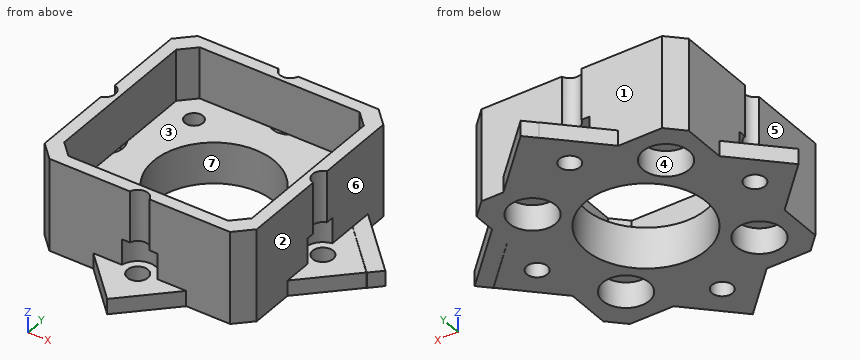
from build123d import *

# Parameters (mm, degrees)
F4_DEPTH  = 18
F2_R      = 1.75
F2_R_2    = 11.75
F5_DEPTH  = 8
F3_R      = 2
F3_R_2    = 1.75
F3_R_3    = 11.75
F6_DEPTH  = 3
F7_DEPTH  = 18
F8_R      = 4.5
F8_R_2    = 1.75
F9_DEPTH  = 5
F10_DEPTH = 5
F11_R     = 3.5
F12_DEPTH = 5
F14_DEPTH = 3
F15_DEPTH = 5
F16_DEPTH = 5
F17_R     = 1.75
F18_DEPTH = 5


with BuildPart() as f4:
    # F1 (on Top) → F4 (new body)
    with BuildSketch(Plane.XY):
        Polygon((-17.5979303911, 20.6482383256), (-20.6482383256, 17.5979303911), (-20.6482383256, -17.5979303911), (-17.5979303911, -20.6482383256), (17.5979303911, -20.6482383256), (20.6482383256, -17.5979303911), (20.6482383256, 17.5979303911), (17.5979303911, 20.6482383256), align=None)
        Polygon((-15.5676494429, -18.266042013), (-18.266042013, -15.5676494429), (-18.266042013, 15.5676494429), (-15.5676494429, 18.266042013), (15.5676494429, 18.266042013), (18.266042013, 15.5676494429), (18.266042013, -15.5676494429), (15.5676494429, -18.266042013), align=None, mode=Mode.SUBTRACT)
    extrude(amount=F4_DEPTH)

    # F2 (on Top) → F5 (join)
    with BuildSketch(Plane.XY):
        Polygon((-15.5676494429, 18.266042013), (-18.266042013, 15.5676494429), (-18.266042013, -15.5676494429), (-15.5676494429, -18.266042013), (15.5676494429, -18.266042013), (18.266042013, -15.5676494429), (18.266042013, 15.5676494429), (15.5676494429, 18.266042013), align=None)
        with Locations((-13, -13)):
            Circle(F2_R, mode=Mode.SUBTRACT)
        with Locations((13, -13)):
            Circle(F2_R, mode=Mode.SUBTRACT)
        with Locations((-13, 13)):
            Circle(F2_R, mode=Mode.SUBTRACT)
        Circle(F2_R_2, mode=Mode.SUBTRACT)
        with Locations((13, 13)):
            Circle(F2_R, mode=Mode.SUBTRACT)
    extrude(amount=F5_DEPTH)

    # F3 (on Top) → F6 (join)
    with BuildSketch(Plane.XY):
        Polygon((-29.6984848098, 0), (0, -29.6984848098), (29.6984848098, 0), (0, 29.6984848098), align=None)
        with Locations((0, -21.2132034356)):
            Circle(F3_R, mode=Mode.SUBTRACT)
        with Locations((-13, -13)):
            Circle(F3_R_2, mode=Mode.SUBTRACT)
        with Locations((13, -13)):
            Circle(F3_R_2, mode=Mode.SUBTRACT)
        with Locations((-21.2132034356, 0)):
            Circle(F3_R, mode=Mode.SUBTRACT)
        Circle(F3_R_3, mode=Mode.SUBTRACT)
        with Locations((-13, 13)):
            Circle(F3_R_2, mode=Mode.SUBTRACT)
        with Locations((0, 21.2132034356)):
            Circle(F3_R, mode=Mode.SUBTRACT)
        with Locations((13, 13)):
            Circle(F3_R_2, mode=Mode.SUBTRACT)
        with Locations((21.2132034356, 0)):
            Circle(F3_R, mode=Mode.SUBTRACT)
    extrude(amount=F6_DEPTH)

    # F3 (on Top) → F7 (cut)
    with BuildSketch(Plane.XY):
        with Locations((21.2132034356, 0)):
            Circle(F3_R)
        with Locations((0, 21.2132034356)):
            Circle(F3_R)
        with Locations((0, -21.2132034356)):
            Circle(F3_R)
        with Locations((-21.2132034356, 0)):
            Circle(F3_R)
    extrude(amount=F7_DEPTH, mode=Mode.SUBTRACT)

    # F8 (on face) + F2 (on Top) → F9 (cut)
    with BuildSketch(Plane(origin=(0, 0, 0), x_dir=(1, 0, 0), z_dir=(0, 0, -1))):
        with Locations((-13, -13)):
            Circle(F8_R)
        with Locations((-13, -13)):
            Circle(F8_R_2, mode=Mode.SUBTRACT)
    with BuildSketch(Plane.XY):
        with Locations((-13, 13)):
            Circle(F2_R)
    extrude(amount=-F9_DEPTH, dir=(0, 0, -1), mode=Mode.SUBTRACT)

    # F8 (on face) + F2 (on Top) → F10 (cut)
    with BuildSketch(Plane(origin=(0, 0, 0), x_dir=(1, 0, 0), z_dir=(0, 0, -1))):
        with Locations((13, 13)):
            Circle(F8_R)
        with Locations((13, 13)):
            Circle(F8_R_2, mode=Mode.SUBTRACT)
    with BuildSketch(Plane.XY):
        with Locations((13, -13)):
            Circle(F2_R)
    extrude(amount=-F10_DEPTH, dir=(0, 0, -1), mode=Mode.SUBTRACT)

    # F11 (on face) → F12 (cut)
    with BuildSketch(Plane.XY.offset(3)):
        with Locations((0, 21.2132034356)):
            Circle(F11_R)
        with Locations((0, -21.2132034356)):
            Circle(F11_R)
        with Locations((21.2132034356, 0)):
            Circle(F11_R)
        with Locations((-21.2132034356, 0)):
            Circle(F11_R)
    extrude(amount=F12_DEPTH, mode=Mode.SUBTRACT)

    # F13 (on face) → F14 (join)
    with BuildSketch(Plane.XY):
        Polygon((13.4627325878, 20.5004686409), (2.1524152157, 31.7889230696), (0.030988478, 29.6674963319), (9.1980161689, 20.5004686409), align=None)
        Polygon((31.875104401, 2.1236881052), (20.4795914376, 13.4971734413), (20.4795914376, 9.2360144303), (29.7514162958, 0), align=None)
    extrude(amount=F14_DEPTH)

    # F8 (on face) → F15 (cut)
    with BuildSketch(Plane(origin=(0, 0, 0), x_dir=(1, 0, 0), z_dir=(0, 0, -1))):
        with Locations((13, -13)):
            Circle(F8_R)
        with Locations((13, -13)):
            Circle(F8_R_2, mode=Mode.SUBTRACT)
    extrude(amount=-F15_DEPTH, mode=Mode.SUBTRACT)

    # F8 (on face) → F16 (cut)
    with BuildSketch(Plane(origin=(0, 0, 0), x_dir=(1, 0, 0), z_dir=(0, 0, -1))):
        with Locations((-13, 13)):
            Circle(F8_R)
        with Locations((-13, 13)):
            Circle(F8_R_2, mode=Mode.SUBTRACT)
    extrude(amount=-F16_DEPTH, mode=Mode.SUBTRACT)

    # F17 (on face) → F18 (cut)
    with BuildSketch(Plane(origin=(19.1230843583, 19.1230843583, 0), x_dir=(-0.7071067812, 0.7071067812, 0), z_dir=(0.7071067812, 0.7071067812, 0))):
        with Locations((33.1568941474, 3.2000013161)):
            Circle(F17_R)
        with Locations((33.1568941474, 16.7999986839)):
            Circle(F17_R)
        with Locations((-33.1568941474, 16.7999986839)):
            Circle(F17_R)
        with Locations((-33.1568941474, 3.2000013161)):
            Circle(F17_R)
    extrude(amount=-F18_DEPTH, mode=Mode.SUBTRACT)


solid = f4.part
Model file for the job. Use its own axes, mm. Face numbers are marked on the shaded views. A direction names the side the tool comes from. Round coordinates to 2 decimals unless told otherwise and drop trailing zeros. Loops run counter-clockwise (first coordinate to the right, second up) from the corner with the lowest first, then second, coordinate; pieces in that order, holes last. Notation, with made-up numbers: M -39.75,39 L -2.75,39 A10 ccw -2.75,48 Z; hole C 25.5,22.25 d4. An arc over 180 degrees is marked long. One line per question, with ' | ' between items.
1) Band-saw the part on B-B (y = -13). Give the cut face in (x, z), then the cut area to 3 significant figures.
Solved:
outline: M -20.65,0 L -17.5,0 L -17.5,5 L -14.75,5 L -14.75,8 L -18.27,8 L -18.27,18 L -20.65,18 Z; M -11.25,5 L -8.5,5 L -8.5,0 L 8.5,0 L 8.5,5 L 11.25,5 L 11.25,8 L -11.25,8 Z; M 14.75,5 L 17.5,5 L 17.5,0 L 20.65,0 L 20.65,18 L 18.27,18 L 18.27,8 L 14.75,8 Z | area: 267 mm²
2) Band-saw the part on C-C (x = 26). Give the cut face in (y, z).
Solved:
outline: M -3.7,0 L 3.7,0 L 3.7,3 L -3.7,3 Z; M 3.74,0 L 7.99,0 L 7.99,3 L 3.74,3 Z
3) Band-saw the part on A-A (z = 12.5). Give the cut face in (x, y).
Solved:
outline: M -20.65,-17.6 L -17.6,-20.65 L -1.92,-20.65 A2 cw 1.92,-20.65 L 17.6,-20.65 L 20.65,-17.6 L 20.65,-1.92 A2 cw 20.65,1.92 L 20.65,17.6 L 17.6,20.65 L 1.92,20.65 A2 cw -1.92,20.65 L -17.6,20.65 L -20.65,17.6 L -20.65,1.92 A2 cw -20.65,-1.92 Z; hole M -18.27,-15.57 L -15.57,-18.27 L 15.57,-18.27 L 18.27,-15.57 L 18.27,15.57 L 15.57,18.27 L -15.57,18.27 L -18.27,15.57 Z
4) Mould opens along X. For the marked faces 5, 6 and 7 say: +X half, -X half, draft (parallel to the pull), parting line (faces both ways), or undercut.
Solved:
face 5: -X half | face 6: +X half | face 7: undercut
5) Flat gauge pins, fed straight in: pin 1 (4.5 mm diameter, centred on x = 10, z = 12, fed in from +Y); pin 2 (5 mm diameter, centred on y = 14, z = 7, fed in from -X); pin 3 (4 mm diameter, centred on x = -20.5, z = 7, fed in from +Y). Where does each tip first touch, or does it go through?
Solved:
pin 1: stops at y = 20.65 | pin 2: stops at x = -20.65 | pin 3: stops at y = 19.75
6) Drill centre lines: line 1 along Y through (x, z) = (-13, 2.25); line 2 along X through (y, z) = (-13, 5.8); line 3 along Y through (x, z) = (0, 1.4). Where is each one in solid material? Low to high.
Solved:
line 1: y = -20.65 to -17.5, -8.5 to 8.5, 17.5 to 20.65 | line 2: x = -20.65 to -14.75, -11.25 to 11.25, 14.75 to 20.65 | line 3: y = -29.7 to -23.21, -19.21 to -11.75, 11.75 to 19.21, 23.21 to 29.7
7) 3-axis set-ups, long thin cutter, end or side, ignore diameter. For the marked faces 1, 2, 3 and 4: which of +Z, -Z, +X, -X, +Y, -Y reach the whole face in a straight line?
Solved:
face 1: +Z, -X, +Y | face 2: +Z, +X, -Y | face 3: +Z | face 4: -Z
